from build123d import *

# Parameters (mm, degrees)
SKETCH1_W                = 20
SKETCH1_H                = 70
SKETCH1_R                = 2.5
SKETCH1_W_2              = 57
SKETCH1_W_3              = 3
BOSS_EXTRUDE1_DEPTH      = 3
SKETCH1_3_W              = 3
SKETCH1_3_H              = 70
BOSS_EXTRUDE2_DEPTH      = 26
SKETCH3_R                = 11.0045
SKETCH3_R_2              = 6
CUT_EXTRUDE2_DEPTH       = 10
FILLET1_R                = 20
BOSS_EXTRUDE4_START      = 26
SKETCH1_4_W              = 20
SKETCH1_4_H              = 70
SKETCH1_4_R              = 2.5
BOSS_EXTRUDE4_DEPTH      = 3
SKETCH4_R                = 6.5
SKETCH4_R_2              = 4
BOSS_EXTRUDE5_DEPTH      = 10
FILLET2_R                = 1
SKETCH3_4_R              = 11.0045
SKETCH3_4_R_2            = 6
BOSS_EXTRUDE7_DEPTH      = 3
FILLET3_R                = 2
M5_CLEARANCE_HOLE1_D     = 5.5
M5_CLEARANCE_HOLE1_DEPTH = 23
M5_CLEARANCE_HOLE2_D     = 5.5


with BuildPart() as part:
    # Sketch1 → Boss-Extrude1 (new body)
    with BuildSketch(Plane(origin=(0, 0, 0), x_dir=(1, 0, 0), z_dir=(0, 1, 0))):
        with Locations((-30, 0)):
            Rectangle(SKETCH1_W, SKETCH1_H)
        with Locations((-30, -17.5)):
            Circle(SKETCH1_R, mode=Mode.SUBTRACT)
        with Locations((-30, 17.5)):
            Circle(SKETCH1_R, mode=Mode.SUBTRACT)
        with Locations((11.5, 0)):
            Rectangle(SKETCH1_W_2, SKETCH1_H)
        with Locations((-18.5, 0)):
            Rectangle(SKETCH1_W_3, SKETCH1_H)
    extrude(amount=BOSS_EXTRUDE1_DEPTH)

    # Sketch1<3> → Boss-Extrude2 (add)
    with BuildSketch(Plane(origin=(0, 0, 0), x_dir=(1, 0, 0), z_dir=(0, 1, 0))):
        with Locations((-18.5, 0)):
            Rectangle(SKETCH1_3_W, SKETCH1_3_H)
    extrude(amount=BOSS_EXTRUDE2_DEPTH)

    # Sketch3 → Cut-Extrude2 (cut)
    with BuildSketch(Plane(origin=(0, 3, 0), x_dir=(1, 0, 0), z_dir=(0, 1, 0))):
        with Locations((14.15, 0)):
            Circle(SKETCH3_R)
        with Locations((14.15, 0)):
            Circle(SKETCH3_R_2)
    extrude(amount=-CUT_EXTRUDE2_DEPTH, mode=Mode.SUBTRACT)

    # Fillet1
    fillet1_edges = [part.edges().sort_by_distance(p)[0] for p in [
        (40, 1.5, -35),
        (40, 1.5, 35),
    ]]
    fillet(fillet1_edges, radius=FILLET1_R)

    # Sketch1<4> → Boss-Extrude4 (add)
    with BuildSketch(Plane(origin=(0, 0, 0), x_dir=(1, 0, 0), z_dir=(0, 1, 0)).offset(BOSS_EXTRUDE4_START)):
        with Locations((-30, 0)):
            Rectangle(SKETCH1_4_W, SKETCH1_4_H)
        with Locations((-30, -17.5)):
            Circle(SKETCH1_4_R, mode=Mode.SUBTRACT)
        with Locations((-30, 17.5)):
            Circle(SKETCH1_4_R, mode=Mode.SUBTRACT)
    extrude(amount=-BOSS_EXTRUDE4_DEPTH)

    # Sketch4 → Boss-Extrude5 (add)
    with BuildSketch(Plane(origin=(0, 3, 0), x_dir=(1, 0, 0), z_dir=(0, 1, 0))):
        with Locations((14.15, -22)):
            Circle(SKETCH4_R)
        with Locations((14.15, -22)):
            Circle(SKETCH4_R_2, mode=Mode.SUBTRACT)
    extrude(amount=BOSS_EXTRUDE5_DEPTH)

    # Fillet2
    fillet2_edges = [part.edges().sort_by_distance(p)[0] for p in [
        (1.5, 3, 35),
        (1.5, 3, -35),
        (-20, 3, 0),
        (-17, 14.5, 35),
        (-17, 3, 0),
        (-17, 26, 0),
        (-17, 14.5, -35),
        (-40, 3, 0),
        (40, 3, 0),
        (34.142135624, 3, -29.142135624),
        (34.142135624, 3, 29.142135624),
        (-40, 23, 0),
        (-40, 26, 0),
        (-40, 0, 0),
    ]]
    fillet(fillet2_edges, radius=FILLET2_R)

    # Sketch3<4> → Boss-Extrude7 (add)
    with BuildSketch(Plane(origin=(0, 3, 0), x_dir=(1, 0, 0), z_dir=(0, 1, 0))):
        with Locations((14.15, 0)):
            Circle(SKETCH3_4_R)
        with Locations((14.15, 0)):
            Circle(SKETCH3_4_R_2, mode=Mode.SUBTRACT)
    extrude(amount=-BOSS_EXTRUDE7_DEPTH)

    # Fillet3
    fillet3_edges = [part.edges().sort_by_distance(p)[0] for p in [
        (7.65, 13, 22),
        (7.65, 3, 22),
    ]]
    fillet(fillet3_edges, radius=FILLET3_R)

    # M5 Clearance Hole1
    with Locations(Plane(origin=(-17, 0, 0), x_dir=(0, 0, -1), z_dir=(1, 0, 0))):
        with Locations((-17.5, 13), (17.5, 13)):
            Hole(M5_CLEARANCE_HOLE1_D / 2, depth=M5_CLEARANCE_HOLE1_DEPTH)

    # M5 Clearance Hole2 (through all)
    with Locations(Plane(origin=(0, 26, 0), x_dir=(1, 0, 0), z_dir=(0, 1, 0))):
        with Locations((-30, -17.5), (-30, 17.5)):
            Hole(M5_CLEARANCE_HOLE2_D / 2)


solid = part.part
Can you work these out from the model? Positions are in its coordinate system, mm. A direction names the side the tool comes from. Coordinates: 2 decimals unless noted, no trailing zeros. Write each loop counter-clockwise with the first axis right and the second up, starting at its lowest first coordinate (ties: lowest second). Pieces come first, ordered by that corner, then holes. Notation, with made-up numbers: M 4.25,19.5 L 45.25,19.5 A22 cw 45.25,26.5 Z; hole C 72.5,59 d8. An arc over 180 degrees is marked long. Use one line per item in the form item = value.
Q1. If we section it at B-B (x = -30): Write out the boundary of the cut face in (y, z), then the cut area to 3 significant figures.
Model answer:
outline = M 0,-35 L 3,-35 L 3,-20.25 L 0,-20.25 Z; M 0,-14.75 L 3,-14.75 L 3,14.75 L 0,14.75 Z; M 0,20.25 L 3,20.25 L 3,35 L 0,35 Z; M 23,-35 L 26,-35 L 26,-20.25 L 23,-20.25 Z; M 23,-14.75 L 26,-14.75 L 26,14.75 L 23,14.75 Z; M 23,20.25 L 26,20.25 L 26,35 L 23,35 Z
area = 354 mm^2
Q2. I need wall thicknesses on line 1 along Z through (x, y) = (-30, 0.75); line 2 along X through (y, z) = (7.5, 22); line 3 along Y through (x, z) = (-18, 17.5). Which ranges of each line are inside material? Lowest first, please. Write a range as from..to.
Model answer:
line_1 = -35..-20.25, -14.75..14.75, 20.25..35
line_2 = -20..-17, 7.65..10.15, 18.15..20.65
line_3 = 0..10.25, 15.75..26
Q3. If we section it at D-D (z = -11.5): Write out the boundary of the cut face in (x, y), then the cut area to 3 significant figures.
Model answer:
outline = M -40,1 A1 ccw -39,0 L 40,0 L 40,2 A1 ccw 39,3 L -16,3 A1 cw -17,4 L -17,25 A1 ccw -18,26 L -39,26 A1 ccw -40,25 L -40,24 A1 ccw -39,23 L -20,23 L -20,4 A1 cw -21,3 L -39,3 A1 ccw -40,2 Z
area = 368 mm^2
Q4. We'd pull the mould along X, two halves only. Please class faces 1 (the cylindrical face through (34.297, 1.014, -28.986)), 2 (the cylindrical face through (-27.253, 1.479, -17.621)), 3 (the cylindrical face through (-18.521, 13.121, -20.247)), 4 (the cylindrical face through (19.873, 1.521, -1.802)): +X half, -X half, draft (parallel to the pull), parting line (faces both ways), or undercut.
Model answer:
face_1 = +X half
face_2 = undercut
face_3 = draft
face_4 = undercut
Q5. For faces 5 (the flat face through (-30, 23, 0)), 6 (the cylindrical face through (-27.253, 24.479, 17.379)), 7 (the cylindrical face through (13.304, 7.958, 15.555)), which set-ups out of +Z, -Z, +X, -X, +Y, -Y let a thin tool reach every point of the face, with its end or its side?
Model answer:
face_5 = +Z, -Z, -X
face_6 = +Y, -Y
face_7 = +Y
Q6. For P1, Ø6.5, axis at y = 13, z = -17.5, coming from the +X side; P2, Ø4.5, axis at y = 13, z = 17.5, coming from the -X side; P3, Ø10, axis at x = 13, z = 22, coming from the +Y side; P4, Ø4.5, axis at x = -30, z = 17.5, coming from the +Y side, each with a flat end and sliding along its axis, tell me the tip position at first contact or that it passes through.
Model answer:
P1 = -17
P2 = 8.36
P3 = 13
P4 = through
Q7. If we section it at A-A (y = 7.75): Write out the boundary of the cut face in (x, z), then the cut area to 3 significant figures.
Model answer:
outline = M -20,-35 L -18,-35 A1 ccw -17,-34 L -17,34 A1 ccw -18,35 L -20,35 Z; C 14.15,22 d13; hole C 14.15,22 d8
area = 292 mm^2
Q8. If we section it at C-C (z = 1): Write out the boundary of the cut face in (x, y).
Model answer:
outline = M -40,1 A1 ccw -39,0 L 8.23,0 L 8.23,3 L -16,3 A1 cw -17,4 L -17,25 A1 ccw -18,26 L -39,26 A1 ccw -40,25 L -40,24 A1 ccw -39,23 L -20,23 L -20,4 A1 cw -21,3 L -39,3 A1 ccw -40,2 Z; M 20.07,0 L 40,0 L 40,2 A1 ccw 39,3 L 20.07,3 Z
